The listing builds one solid part. Answer for the finished solid, in the listing's coordinates (mm). A direction names the side the tool comes from. Round coordinates to 2 decimals unless told otherwise and drop trailing zeros. Write each loop counter-clockwise with the first axis right and the second up, starting at its lowest first coordinate (ties: lowest second). Pieces come first, ordered by that corner, then holes.
Item 1: Find the intervals of material crossed by probe 1 along Y at (x, z) = (18.75, 2.05); probe 2 along Y at (x, z) = (2.25, 1.95); probe 3 along X at (y, z) = (16.75, 0.15), in increasing order.
Item 2: A tool of negligible diameter and unlimited length cuts with its end or side. For faces 1 (the face through (21, 13.5, 1)), 2 (the face through (21, 3.5, 1)), 3 (the face through (28, 8, 1)), from which of +Z, -Z, +X, -X, +Y, -Y can it reach the whole face along a straight path? Write none if from no direction.
Item 3: Each of these flat-tipped pins is pushed along its axis until it touches: pin 1 (0.9 mm diameter, centred on x = 22.5, z = 1.5, fed in from +Y); pin 2 (1 mm diameter, centred on x = 15, z = 1.5, fed in from -Y). Where does it stop, or does it pass through?
Item 4: Find section B-B on x = 22.5. Give the vertices of the cut face in (y, z).
Item 5: Find section C-C on y = 12.75. Give the vertices of the cut face in (x, z).
```python
from build123d import *

# Parameters (mm, degrees)
F1_DEPTH = 3
F2_R     = 3.49999
F3_R     = 3.49999


# Not quite as in the source:
# - a fillet or chamfer is up to 0.001 mm smaller than in the source, because OpenCascade refuses the exact size


with BuildPart() as f1:
    # F0 (on Top) → F1 (new body)
    with BuildSketch(Plane.XY):
        Polygon((0, 12), (0, 0), (10, 0), (10, 3.5), (28, 3.5), (28, 13.5), (10, 13.5), (10, 17), (5, 17), align=None)
    extrude(amount=F1_DEPTH)

    # F2 (radius 3.5 in the source; OpenCascade refuses exactly that, so slightly less here)
    f2_edges = [f1.edges().sort_by_distance(p)[0] for p in [
        (10, 13.5, 1.5),
    ]]
    fillet(f2_edges, radius=F2_R)

    # F3 (radius 3.5 in the source; OpenCascade refuses exactly that, so slightly less here)
    f3_edges = [f1.edges().sort_by_distance(p)[0] for p in [
        (10, 3.5, 1.5),
    ]]
    fillet(f3_edges, radius=F3_R)


solid = f1.part
```
Check values:
1. probe 1: y = 3.5 to 13.5
1. probe 2: y = 0 to 14.25
1. probe 3: x = 4.75 to 10.01
2. face 1: +Z, -Z, +X, +Y
2. face 2: +Z, -Z, +X, -Y
2. face 3: +Z, -Z, +X, +Y, -Y
3. pin 1: stops at y = 13.5
3. pin 2: stops at y = 3.5
4. outline: (3.5, 0) - (13.5, 0) - (13.5, 3) - (3.5, 3) - close
5. outline: (0.75, 0) - (28, 0) - (28, 3) - (0.75, 3) - close
